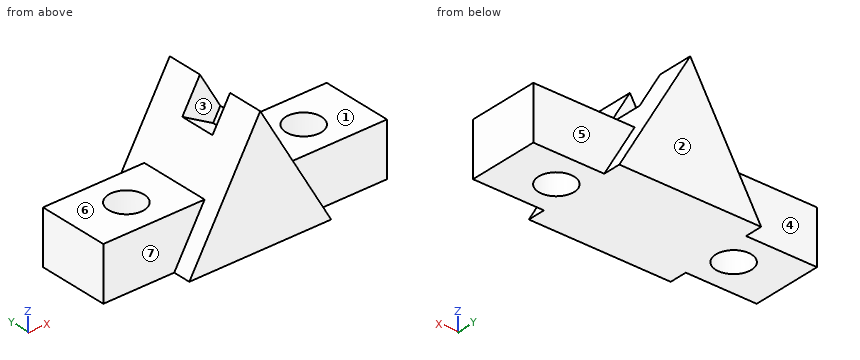
```python
from build123d import *

# Parameters (mm, degrees)
F0_W      = 2032
F0_H      = 889
F1_DEPTH  = 762
F3_DEPTH  = 127
F5_DEPTH  = 762
F7_DEPTH  = 889
F9_DEPTH  = 762
F11_DEPTH = 127
F12_W     = 254
F12_H     = 254
F13_DEPTH = 254
F15_DEPTH = 381
F17_DEPTH = 381
F18_R     = 127
F19_DEPTH = 381
F20_R     = 127
F21_DEPTH = 381
F22_R     = 127
F23_DEPTH = 381
F24_W     = 254
F24_H     = 254
F25_DEPTH = 254


with BuildPart() as f1:
    # F0 (on Front) → F1 (new body)
    with BuildSketch(Plane.XZ):
        with Locations((-1016, 444.5)):
            Rectangle(F0_W, F0_H)
    extrude(amount=F1_DEPTH)

    # F2 (on face) → F3 (cut)
    with BuildSketch(Plane.XZ.offset(762)):
        Polygon((-725.7142857143, 381), (-508, 0), (0, 0), (0, 381), align=None)
        Polygon((-2032, 381), (-2032, 0), (-1524, 0), (-1306.2857142857, 381), align=None)
    extrude(amount=-F3_DEPTH, mode=Mode.SUBTRACT)

    # F4 (on face) → F5 (join)
    with BuildSketch(Plane.XZ.offset(762)):
        Polygon((-2032, 381), (-1306.2857142857, 381), (-1016, 889), (-2032, 889), align=None)
        Polygon((0, 889), (-1016, 889), (-725.7142857143, 381), (0, 381), align=None)
    extrude(amount=-F5_DEPTH)

    # F6 (on face) → F7 (cut)
    with BuildSketch(Plane.XZ.offset(762)):
        Polygon((-2032, 381), (-1306.2857142857, 381), (-1016, 889), (-2032, 889), align=None)
    extrude(amount=-F7_DEPTH, mode=Mode.SUBTRACT)

    # F8 (on face) → F9 (cut)
    with BuildSketch(Plane.XZ.offset(762)):
        Polygon((-1016, 889), (-725.7142857143, 381), (0, 381), (0, 889), align=None)
    extrude(amount=-F9_DEPTH, mode=Mode.SUBTRACT)

    # F10 (on face) → F11 (cut)
    with BuildSketch(Plane(origin=(0, 0, 0), x_dir=(-1, 0, 0), z_dir=(0, 1, 0))):
        Polygon((0, 381), (0, 0), (508, 0), (725.7142857143, 381), align=None)
        Polygon((1306.2857142857, 381), (1524, 0), (2032, 0), (2032, 381), align=None)
    extrude(amount=-F11_DEPTH, mode=Mode.SUBTRACT)

    # F12 (on face) → F13 (cut)
    with BuildSketch(Plane(origin=(-382.9538461538, 0, -218.8307692308), x_dir=(0, 1, 0), z_dir=(0.8682431421, 0, 0.4961389384))):
        with Locations((-381, 1148.9453147192)):
            Rectangle(F12_W, F12_H)
    extrude(amount=F13_DEPTH, mode=Mode.SUBTRACT)

    # F14 (on face) → F15 (cut)
    with BuildSketch(Plane.XY.offset(381)):
        with BuildLine():
            ThreePointArc((-1524, -381), (-1561.1974387893, -291.1974387893), (-1651, -254))
            Line((-1651, -254), (-1651, -381))
            Line((-1651, -381), (-1778, -381))
            ThreePointArc((-1778, -381), (-1651, -508), (-1524, -381))
        make_face()
        with BuildLine():
            Line((-1651, -381), (-1651, -254))
            ThreePointArc((-1651, -254), (-1740.8025612107, -291.1974387893), (-1778, -381))
            Line((-1778, -381), (-1651, -381))
        make_face()
    extrude(amount=-F15_DEPTH, mode=Mode.SUBTRACT)

    # F16 (on face) → F17 (join)
    with BuildSketch(Plane.XY.offset(381)):
        with BuildLine():
            ThreePointArc((-254, -381), (-291.1974387893, -291.1974387893), (-381, -254))
            Line((-381, -254), (-381, -381))
            Line((-381, -381), (-254, -381))
        make_face()
        with BuildLine():
            Line((-381, -381), (-381, -254))
            ThreePointArc((-381, -254), (-470.8025612107, -470.8025612107), (-254, -381))
            Line((-254, -381), (-381, -381))
        make_face()
    extrude(amount=-F17_DEPTH)

    # F18 (on face) → F19 (join)
    with BuildSketch(Plane.XY.offset(381)):
        with Locations((-381, -381)):
            Circle(F18_R)
    extrude(amount=-F19_DEPTH)

    # F20 (on face) → F21 (cut)
    with BuildSketch(Plane.XY.offset(381)):
        with Locations((-381, -381)):
            Circle(F20_R)
    extrude(amount=F21_DEPTH, mode=Mode.SUBTRACT)

    # F22 (on face) → F23 (cut)
    with BuildSketch(Plane.XY.offset(381)):
        with Locations((-381, -381)):
            Circle(F22_R)
    extrude(amount=-F23_DEPTH, mode=Mode.SUBTRACT)

    # F24 (on face) → F25 (cut)
    with BuildSketch(Plane(origin=(-1148.8615384615, 0, 656.4923076923), x_dir=(0, -1, 0), z_dir=(-0.8682431421, 0, 0.4961389384))):
        with Locations((381, 140.7909919781)):
            Rectangle(F24_W, F24_H)
        with Locations((381, 394.7909919781)):
            Rectangle(F24_W, F24_H)
    extrude(amount=-F25_DEPTH, mode=Mode.SUBTRACT)


solid = f1.part
```
The listing builds one solid part. Answer for the finished solid, in the listing's coordinates (mm). Face numbers are marked on the shaded views. A direction names the side the tool comes from. Coordinates: 2 decimals unless noted, no trailing zeros. Write each loop counter-clockwise with the first axis right and the second up, starting at its lowest first coordinate (ties: lowest second). Pieces come first, ordered by that corner, then holes. Notation, with made-up numbers: (-34.5, 69.25) - (6.5, 69.25) arc R22 ccw to (6.5, 77.25) - close; hole circle Ø2 at (26, 70). An arc over 180 degrees is marked (long way). One line per item, written item: value.
1) A tool of negligible diameter and unlimited length cuts with its end or side. For the marked faces 4, 5, 6 and 7, from which of +Z, -Z, +X, -X, +Y, -Y can it reach the whole face along a straight path? Write none if from no direction.
Geometry check:
face 4: +Z, -X, +Y
face 5: +Z, +X, +Y
face 6: +Z, -X, +Y, -Y
face 7: +Z, -X, -Y
2) Consider line 1 along Y through (x, z) = (-958, 654.5); line 2 along X through (y, z) = (-464, 83); line 3 along Y through (x, z) = (-1651, 207). Determine where each line is inside the solid, lowest interval first. Write a range as from..to.
Geometry check:
line 1: y = -762..-508, -254..0
line 2: x = -2032..-1747.12, -1554.88..-477.12, -284.88..0
line 3: y = -635..-508, -254..-127
3) Find section D-D (z = 831). Give the vertices of the cut face in (x, y).
Geometry check:
outline: (-1049.14, -762) - (-982.86, -762) - (-982.86, -508) - (-1049.14, -508) - close; (-1049.14, -254) - (-982.86, -254) - (-982.86, 0) - (-1049.14, 0) - close
4) For a pull along Y with two mould halves and no side action, classify the marked faces 1, 2 and 3 as pulls with the +Y half, pulls with the -Y half, needs draft (parallel to the pull), parting line crosses it, or undercut.
Geometry check:
face 1: needs draft
face 2: pulls with the +Y half
face 3: undercut
5) Each of these flat-tipped pins is pushed along its axis until it touches: pin 1 Ø4 at (y, z) = (-77, 466.5) entering from -X; pin 2 Ø2 at (x, y) = (-862, -249) entering from +Z; pin 3 Ø12 at (x, z) = (-1446, 377) entering from -Y. Where does it stop, or does it pass through?
Geometry check:
pin 1: stops at x = -1258.57
pin 2: stops at z = 621.25
pin 3: stops at y = -635
6) Find section B-B (y = -381). Give the vertices of the cut face in (x, z), and give its area (3 significant figures).
Geometry check:
outline: (-2032, 0) - (-1778, 0) - (-1778, 381) - (-2032, 381) - close; (-1524, 0) - (-508, 0) - (-508, 381) - (-725.71, 381) - (-869.73, 633.02) - (-921.49, 542.45) - (-1142.02, 668.47) - (-1306.29, 381) - (-1524, 381) - close; (-254, 0) - (0, 0) - (0, 381) - (-254, 381) - close
area: 683,000 mm2
7) Find section C-C (x = -381). Give the vertices of the cut face in (y, z), and give its area (3 significant figures).
Geometry check:
outline: (-635, 0) - (-508, 0) - (-508, 381) - (-635, 381) - close; (-254, 0) - (-127, 0) - (-127, 381) - (-254, 381) - close
area: 96,800 mm2
8) Find section A-A (z = 175). Give the vertices of the cut face in (x, y), and give its area (3 significant figures).
Geometry check:
outline: (-2032, -635) - (-1424, -635) - (-1424, -762) - (-608, -762) - (-608, -635) - (0, -635) - (0, -127) - (-608, -127) - (-608, 0) - (-1424, 0) - (-1424, -127) - (-2032, -127) - close; hole circle Ø254 at (-1651, -381); hole circle Ø254 at (-381, -381)
area: 1,140,000 mm2
